The model under review builds one solid part; all positions refer to its coordinate system, in mm. A direction names the side the tool comes from. Coordinates: 2 decimals unless noted, no trailing zeros. Write each loop counter-clockwise with the first axis right and the second up, starting at its lowest first coordinate (ties: lowest second). Pieces come first, ordered by that corner, then holes.
```python
from build123d import *

# Parameters (mm, degrees)
ESQUISSE1_R                  = 160
ESQUISSE1_R_2                = 110
BOSS_EXTRU_1_DEPTH           = 10
ESQUISSE2_W                  = 10.3
ESQUISSE2_H                  = 31.7
ENL_V_MAT_EXTRU_2_DEPTH      = 10
ESQUISSE3_R                  = 6
ENL_V_MAT_EXTRU_3_DEPTH      = 11
R_P_TITION_CIRCULAIRE1_COUNT = 10
R_P_TITION_CIRCULAIRE2_COUNT = 5


with BuildPart() as part:
    # Esquisse1 → Boss.-Extru.1 (new body)
    with BuildSketch(Plane(origin=(0, 0, 0), x_dir=(1, 0, 0), z_dir=(0, 1, 0))):
        with Locations(Location((0, 0, 0), (0, 0, 270))):  # turned: the seam where the file's is
            Circle(ESQUISSE1_R)
        with Locations(Location((0, 0, 0), (0, 0, 270))):  # turned: the seam where the file's is
            Circle(ESQUISSE1_R_2, mode=Mode.SUBTRACT)
    extrude(amount=BOSS_EXTRU_1_DEPTH)

    # Esquisse2 → Enl_v. mat.-Extru.2 (cut)
    with BuildSketch(Plane(origin=(0, 10, 0), x_dir=(1, 0, 0), z_dir=(0, 1, 0))):
        with Locations((0, -144.15)):
            Rectangle(ESQUISSE2_W, ESQUISSE2_H)
    enl_v_mat_extru_2 = extrude(amount=-ENL_V_MAT_EXTRU_2_DEPTH, mode=Mode.SUBTRACT)

    # Esquisse3 → Enl_v. mat.-Extru.3 (cut, through all)
    with BuildSketch(Plane(origin=(0, 10, 0), x_dir=(1, 0, 0), z_dir=(0, 1, 0))):
        with Locations(Location((-41.099260252, -126.490516667, 0), (0, 0, 270))):  # turned: the seam where the file's is
            Circle(ESQUISSE3_R)
    enl_v_mat_extru_3 = extrude(amount=-ENL_V_MAT_EXTRU_3_DEPTH, mode=Mode.SUBTRACT)

    # R_p_tition circulaire1: Enl_v. mat.-Extru.2 ×10 about axis
    r_p_tition_circulaire1_axis = Axis((0, 0, 0), (0, 1, 0))
    for i in range(1, R_P_TITION_CIRCULAIRE1_COUNT):
        add(enl_v_mat_extru_2.rotate(r_p_tition_circulaire1_axis, i * 360 / R_P_TITION_CIRCULAIRE1_COUNT), mode=Mode.SUBTRACT)

    # R_p_tition circulaire2: Enl_v. mat.-Extru.3 ×5 about axis
    r_p_tition_circulaire2_axis = Axis((0, 0, 0), (0, 1, 0))
    for i in range(1, R_P_TITION_CIRCULAIRE2_COUNT):
        add(enl_v_mat_extru_3.rotate(r_p_tition_circulaire2_axis, i * 360 / R_P_TITION_CIRCULAIRE2_COUNT), mode=Mode.SUBTRACT)


solid = part.part
```
Item 1: To check wall thickness, follow line 1 along X through (y, z) = (4.75, 0); line 2 along Z through (x, y) = (-136.5, 7); line 3 along X through (y, z) = (3, -78). State the ranges of each line that lie inside material, in increasing order.
Solved:
line 1: x = -160 to -139, -127 to -110, 110 to 160
line 2: z = -83.47 to -49.77, -38.94 to -4.87, 4.87 to 38.94, 49.77 to 83.47
line 3: x = -139.7 to -77.56, 77.56 to 101.6, 113.6 to 139.7
Item 2: Take a section at B-B, the plane z = 17. Write out the cut boundary in (x, y).
Solved:
outline: (-159.09, 0) - (-108.68, 0) - (-108.68, 10) - (-159.09, 10) - close; (108.68, 0) - (159.09, 0) - (159.09, 10) - (108.68, 10) - close
Item 3: Take a section at A-A, the plane x = 0. Write out the cut boundary in (y, z).
Solved:
outline: (0, -128.3) - (10, -128.3) - (10, -110) - (0, -110) - close; (0, 110) - (10, 110) - (10, 128.3) - (0, 128.3) - close
Item 4: Take a section at D-D, the plane y = 4. Count the separate pieces of the cut face and the enclosed holes in it, plus the area to 3 significant figures.
Solved:
separate pieces: 1
enclosed holes: 6
area: 38,600 mm2
Item 5: Mouldability with a two-part tool opening along X and no side actions: class faces 1 (the face through (75.355, 5.07, 103.839)), 2 (the face through (50.043, 4.93, -151.973)), 3 (the face through (-104, 10, -38)) as pulls with the +X half, pulls with the -X half, needs draft (parallel to the pull), parting line crosses it, or undercut.
Solved:
face 1: undercut
face 2: pulls with the +X half
face 3: needs draft
Item 6: Machinability: for faces 4 (the face through (-129.07, 4.93, -94.556)), 5 (the face through (-5.15, 5, -144)), 6 (the face through (138.857, 5.07, -39.702)), 7 (the face through (-5.15, 5, 144)), which of the approach directions +Z, -Z, +X, -X, +Y, -Y give a long, thin tool a straight path to every point of the face, cutting with its end or side? Answer none if there is none.
Solved:
face 4: -Z, -X, +Y, -Y
face 5: -Z, +Y, -Y
face 6: +Y, -Y
face 7: +Z, +Y, -Y
Item 7: Take a section at C-C, the plane x = -132.5. Write out the cut boundary in (y, z).
Solved:
outline: (0, -89.69) - (10, -89.69) - (10, -48.47) - (0, -48.47) - close; (0, -37.64) - (10, -37.64) - (10, -5.98) - (0, -5.98) - close; (0, 5.98) - (10, 5.98) - (10, 37.64) - (0, 37.64) - close; (0, 48.47) - (10, 48.47) - (10, 89.69) - (0, 89.69) - close
Item 8: For pin 1 (2 mm diameter, centred on y = 2, z = -119.5, fed in from +X); pin 2 (3 mm diameter, centred on y = 3.5, z = 142.5, fed in from -X); pin 3 (2 mm diameter, centred on x = 21, y = 1.5, fed in from +Z); pin 4 (11 mm diameter, centred on x = -41.1, z = 126.49, fed in from -Y), all flat-tipped, find the tip position at first contact; note any pin that passes through.
Solved:
pin 1: stops at x = 107.51
pin 2: stops at x = -75.62
pin 3: stops at z = 158.75
pin 4: passes through
